For this review, take the finished solid that the model builds, in its own axes (mm). Face numbers are marked on the shaded views. A direction names the side the tool comes from. Round coordinates to 2 decimals unless told otherwise and drop trailing zeros. Order: outer loops, then holes, each group sorted by start corner. A loop starts at its lowest first (then second) coordinate and runs counter-clockwise, first axis right, second up. Notation, with made-up numbers: M 36,-31 L 63,-31 A5 ccw 63,-24 Z; hole C 49.25,-20 d9. An arc over 180 degrees is marked long. Use a Markdown table: item, result.
from build123d import *

# Parameters (mm, degrees)
EXTRUDE_1_DEPTH          = 6
EXTRUDE_START            = -3.991967
EXTRUDE_2_DEPTH          = 3.991967
PATTERN_CIRCULAR_1_COUNT = 3
PATTERN_CIRCULAR_1_ANGLE = 90
SKETCH_4_R               = 3
CUT_EXTRUDE_1_DEPTH      = 7.0000001


with BuildPart() as part:
    # Sketch 1 → Extrude 1 (new body)
    with BuildSketch(Plane.XY):
        with BuildLine():
            Line((-4.5, 0), (-4.5, -18.2))
            Line((-4.5, -18.2), (-3, -18.2))
            Line((-3, -18.2), (-3, -14.6))
            ThreePointArc((-3, -14.6), (-1.968245837, -12.85), (-3, -11.1))
            Line((-3, -11.1), (-3, -10))
            Line((-3, -10), (3, -10))
            Line((3, -10), (3, -11.1))
            ThreePointArc((3, -11.1), (1.968245837, -12.85), (3, -14.6))
            Line((3, -14.6), (3, -18.2))
            Line((3, -18.2), (4.5, -18.2))
            Line((4.5, -18.2), (4.5, 0))
            ThreePointArc((4.5, 0), (0, 4.5), (-4.5, 0))
        make_face()
    extrude_1 = extrude(amount=EXTRUDE_1_DEPTH)

    # Sketch 3 → Extrude 2 (add)
    with BuildSketch(Plane.XZ.offset(18.2).offset(EXTRUDE_START)):
        with BuildLine():
            Line((-3, 6), (-3, 0))
            Line((-3, 0), (-2.5, 1))
            Line((-2.5, 1), (-2.5, 1.5))
            ThreePointArc((-2.5, 1.5), (-2.757359313, 3), (-2.5, 4.5))
            Line((-2.5, 4.5), (-2.5, 5))
            Line((-2.5, 5), (-3, 6))
        make_face()
        with BuildLine():
            Line((3, 0), (2.5, 1))
            Line((2.5, 1), (2.5, 1.5))
            ThreePointArc((2.5, 1.5), (2.757359313, 3), (2.5, 4.5))
            Line((2.5, 4.5), (2.5, 5))
            Line((2.5, 5), (3, 6))
            Line((3, 6), (3, 0))
        make_face()
    extrude_2 = extrude(amount=EXTRUDE_2_DEPTH)

    # Pattern Circular 1: Extrude 1, Extrude 2 ×3 about axis
    pattern_circular_1_axis = Axis((0, 0, 0), (0, 0, 1))
    for i in range(1, PATTERN_CIRCULAR_1_COUNT):
        add(extrude_1.rotate(pattern_circular_1_axis, i * PATTERN_CIRCULAR_1_ANGLE / (PATTERN_CIRCULAR_1_COUNT - 1)))
        add(extrude_2.rotate(pattern_circular_1_axis, i * PATTERN_CIRCULAR_1_ANGLE / (PATTERN_CIRCULAR_1_COUNT - 1)))

    # Sketch 4 → Cut-Extrude 1 (cut, through all)
    with BuildSketch(Plane.XY.offset(6)):
        Circle(SKETCH_4_R)
        with BuildLine():
            Line((8.75, 3), (3.354101966, 3))
            ThreePointArc((3.354101966, 3), (4.378625055, 1.038095674), (4.343906601, -1.174936357))
            Line((4.343906601, -1.174936357), (8.75, -3))
            Line((8.75, -3), (8.75, 3))
        make_face()
        with BuildLine():
            Line((3, -8.75), (1.174936357, -4.343906601))
            ThreePointArc((1.174936357, -4.343906601), (-1.038095674, -4.378625055), (-3, -3.354101966))
            Line((-3, -3.354101966), (-3, -8.75))
            Line((-3, -8.75), (3, -8.75))
        make_face()
        with BuildLine():
            Line((8.308504679, -4.065863992), (4.065863992, -8.308504679))
            Line((4.065863992, -8.308504679), (2.240800349, -3.90241128))
            ThreePointArc((2.240800349, -3.90241128), (3.181980515, -3.181980515), (3.90241128, -2.240800349))
            Line((3.90241128, -2.240800349), (8.308504679, -4.065863992))
        make_face()
    extrude(amount=-CUT_EXTRUDE_1_DEPTH, mode=Mode.SUBTRACT)


solid = part.part
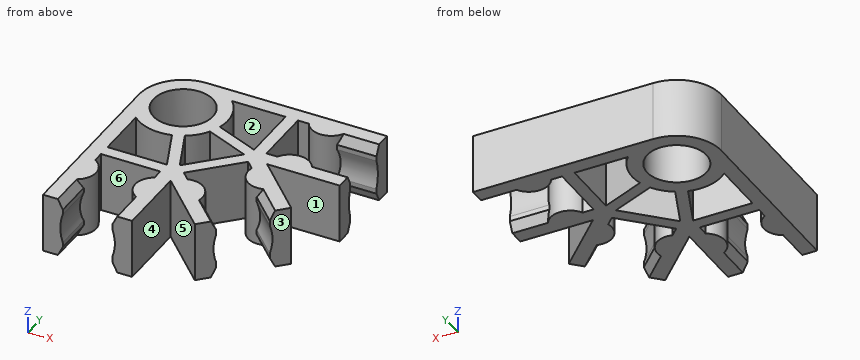
Q1. Machinability: for the marked faces 1, 2 and 3, which of the approach directions +Z, -Z, +X, -X, +Y, -Y give a long, thin tool a straight path to every point of the face, cutting with its end or side? Answer none if there is none.
Determined:
| item | result |
|---|---|
| face 1 | +Z, -Z, +X |
| face 2 | +Z, -Z |
| face 3 | +Z, -Z, +X, -Y |
Q2. Add section B-B (y = -7). Write out the cut boundary in (x, z).
Determined:
| item | result |
|---|---|
| outline | M -4.5,0 L -3,0 L -3,6 L -4.5,6 Z; M 2.28,0 L 3.52,0 L 3.52,6 L 2.28,6 Z; M 5.37,0 L 7.14,0 L 7.14,6 L 5.37,6 Z; M 10.03,0 L 13.36,0 L 13.36,6 L 10.03,6 Z |
Q3. Add section C-C (z = 2.5). Give the number of separate pieces and of enclosed holes in the cut face, then the cut area to 3 significant figures.
Determined:
| item | result |
|---|---|
| separate pieces | 1 |
| enclosed holes | 4 |
| area | 191 mm^2 |
Q4. Add section A-A (y = 0.75). Write out the cut boundary in (x, z), then the cut area to 3 significant figures.
Determined:
| item | result |
|---|---|
| outline | M -4.44,0 L -2.9,0 L -2.9,6 L -4.44,6 Z; M 2.9,0 L 4.44,0 L 4.44,6 L 2.9,6 Z; M 8.75,0 L 10,0 L 10,6 L 8.75,6 Z |
| area | 25.9 mm^2 |
Q5. Clearance check with flat-ended pins moving along their axes: pin 1 (0.5 mm diameter, centred on x = 10.5, z = 2.5, fed in from -Y); pin 2 (1.8 mm diameter, centred on x = 1.5, z = 4, fed in from -Y). State where each tip first meets the part, or that it passes through.
Determined:
| item | result |
|---|---|
| pin 1 | stops at y = -15.49 |
| pin 2 | stops at y = -14.09 |
Q6. Wall thickness on line 1 along X through (y, z) = (-5.5, 5.5); line 2 along X through (y, z) = (-8, 1.5); line 3 along Y through (x, z) = (-1.5, 2): over which ranges is each line inside the solid? List them lowest first. Write a range as [from, to].
Determined:
| item | result |
|---|---|
| line 1 | x = [-4.5, -3], [1.65, 2.9], [6.87, 8.64], [9.74, 11.86] |
| line 2 | x = [-4.5, -3], [2.69, 3.94], [4.37, 6.14], [10.87, 14.36] |
| line 3 | y = [-10, -8.75], [-4.24, -2.6], [2.6, 4.24] |
Q7. Draft analysis for pull direction Y (two halves, no side actions). For the marked faces 4, 5 and 6, state which applies: pulls with the +Y half, pulls with the -Y half, needs draft (parallel to the pull), parting line crosses it, or undercut.
Determined:
| item | result |
|---|---|
| face 4 | needs draft |
| face 5 | pulls with the -Y half |
| face 6 | undercut |
